For this review, take the finished solid that the model builds, in its own axes (mm). Face numbers are marked on the shaded views. A direction names the side the tool comes from. Coordinates: 2 decimals unless noted, no trailing zeros. Loops run counter-clockwise (first coordinate to the right, second up) from the corner with the lowest first, then second, coordinate; pieces in that order, holes last.
1. Take a section at A-A, the plane y = -21. State the section outline as (x, z) points, then the cut area to 3 significant figures.
2. Machinability: for the marked faces 1 and 2, which of the approach directions +Z, -Z, +X, -X, +Y, -Y give a long, thin tool a straight path to every point of the face, cutting with its end or side? Answer none if there is none.
3. Take a section at C-C, the plane x = -65. State the section outline as (y, z) points, then the cut area to 3 significant figures.
4. Mouldability with a two-part tool opening along X and no side actions: class the marked faces 3, 4 and 5 as pulls with the +X half, pulls with the -X half, needs draft (parallel to the pull), parting line crosses it, or undercut.
5. Take a section at B-B, the plane z = -44. State the section outline as (x, y) points.
6. Take a section at D-D, the plane x = 13.5. State the section outline as (y, z) points.
7. To check wall thickness, follow probe 1 along Z at (x, y) = (37.5, -7); probe 2 along X at (y, z) = (-22, -22); probe 3 along X at (y, z) = (-1.5, -12). State the ranges of each line that lie inside material, in increasing order.
8. Clearance check with flat-ended pins moving along their axes: P1, Ø10, axis at x = 58, y = -18, coming from the +Z side; P2, Ø3, axis at x = -46.5, y = -4.5, coming from the -Z side; P3, Ø1.5, axis at y = -13, z = 29, coming from the -X side. State where each tip first meets the part, or that it passes through.
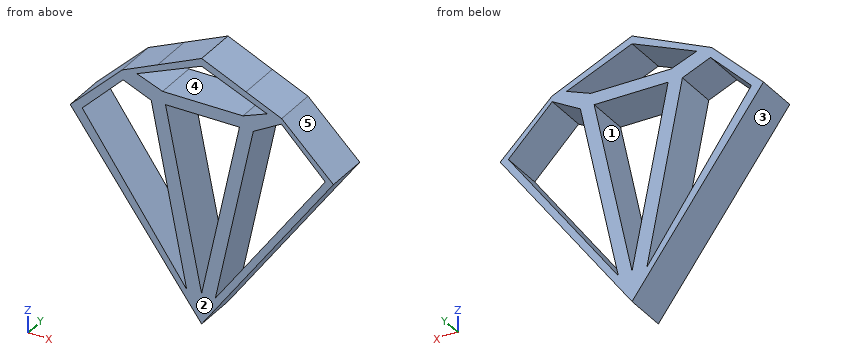
```python
from build123d import *

# Parameters (mm, degrees)
F3_DEPTH = 25.4
F4_DEPTH = 30.48
F7_DEPTH = 50.8


with BuildPart() as f3:
    # F0 (on Front) → F3 (new body)
    with BuildSketch(Plane.XZ):
        Polygon((-75.71096, 26.988449), (0, -76.188624), (-25.316598, 47.161441), (-45.85648, 55.885422), align=None)
        Polygon((26.625417, 47.161441), (0, -76.188624), (75.949796, 26.988449), (46.100167, 55.885422), align=None)
        Polygon((-25.316598, 47.161441), (0, -76.188624), (26.625417, 47.161441), align=None)
        Polygon((-45.85648, 55.885422), (-25.316598, 47.161441), (-15.569561, 60.743305), (-25.316598, 65.086543), align=None)
        Polygon((-15.569561, 60.743305), (16.001999, 60.743305), (25.57465, 65.031505), (0, 76.42746), (-25.316598, 65.086543), align=None)
        Polygon((16.001999, 60.743305), (26.625417, 47.161441), (46.100167, 55.885422), (25.57465, 65.031505), align=None)
        Polygon((-25.316598, 47.161441), (26.625417, 47.161441), (16.001999, 60.743305), (-15.569561, 60.743305), align=None)
    extrude(amount=F3_DEPTH)

    # F1 (on Front) + F2 (on Front) → F4 (cut)
    with BuildSketch(Plane.XZ):
        Polygon((-68.764952, 27.100321), (-8.573943, -58.959331), (-29.023757, 43.573789), (-45.213196, 50.390389), align=None)
        Polygon((71.237154, 27.100321), (45.95891, 52.662592), (29.769467, 43.573789), (7.899523, -58.959331), align=None)
    with BuildSketch(Plane.XZ):
        Polygon((21.816764, 43.573789), (-20.787027, 43.573789), (0, -58.675308), align=None)
        Polygon((0, 71.976312), (-37.260491, 56.354925), (-22.491178, 50.67442), (23.804942, 50.67442), (37.722178, 56.070898), align=None)
    extrude(amount=F4_DEPTH, mode=Mode.SUBTRACT)

    # F5 (on Front) + F6 (on Front) → F7 (cut)
    with BuildSketch(Plane.XZ):
        Polygon((-33.284139, 39.881457), (-44.929173, 44.993915), (-62.822767, 26.248246), (-17.946774, -37.373412), align=None)
    with BuildSketch(Plane.XZ):
        Polygon((16.420284, 39.029382), (-15.390549, 39.029382), (0, -39.361589), align=None)
        Polygon((64.420559, 26.816297), (44.822805, 46.698064), (33.177774, 39.029382), (16.420284, -39.361589), align=None)
    extrude(amount=F7_DEPTH, mode=Mode.SUBTRACT)


solid = f3.part
```
Results list:
1. outline: (-75.71, 26.99) - (0, -76.19) - (75.95, 26.99) - (46.1, 55.89) - (0, 76.43) - (-45.86, 55.89) - close; hole (-68.76, 27.1) - (-8.57, -58.96) - (-29.02, 43.57) - (-45.21, 50.39) - close; hole (-37.26, 56.35) - (-22.49, 50.67) - (23.8, 50.67) - (37.72, 56.07) - (0, 71.98) - close; hole (-20.79, 43.57) - (0, -58.68) - (21.82, 43.57) - close; hole (7.9, -58.96) - (71.24, 27.1) - (45.96, 52.66) - (29.77, 43.57) - close
1. area: 4,080 mm2
2. face 1: +Y, -Y
2. face 2: +Z, -Z, +X, -X, -Y
3. outline: (-25.4, 12.39) - (0, 12.39) - (0, 21.72) - (-25.4, 21.72) - close; (-25.4, 30.82) - (0, 30.82) - (0, 37.36) - (-25.4, 37.36) - close
3. area: 403 mm2
4. face 3: pulls with the -X half
4. face 4: undercut
4. face 5: pulls with the +X half
5. outline: (-23.62, -25.4) - (-19.04, -25.4) - (-19.04, 0) - (-23.62, 0) - close; (-11.56, -25.4) - (-2.98, -25.4) - (-2.98, 0) - (-11.56, 0) - close; (3.13, -25.4) - (11.09, -25.4) - (11.09, 0) - (3.13, 0) - close; (18.91, -25.4) - (23.69, -25.4) - (23.69, 0) - (18.91, 0) - close
6. outline: (-25.4, -57.85) - (0, -57.85) - (0, -51.35) - (-25.4, -51.35) - close; (-25.4, -32.7) - (0, -32.7) - (0, 4.6) - (-25.4, 4.6) - close; (-25.4, 43.57) - (0, 43.57) - (0, 50.67) - (-25.4, 50.67) - close; (-25.4, 66.28) - (0, 66.28) - (0, 70.41) - (-25.4, 70.41) - close
7. probe 1: z = -25.25 to -18.74, 47.91 to 55.98, 56.16 to 59.72
7. probe 2: x = -39.76 to -34.42, -15.95 to -7.46, 7.83 to 15.78, 35.1 to 39.89
7. probe 3: x = -47.1 to -41.42, -17.94 to -9.49, 9.96 to 17.92, 42.46 to 47.25
8. P1: stops at z = 49.21
8. P2: stops at z = -14.86
8. P3: stops at x = -74.41
